Check sheet for the drawn part. Datum: minimum x, y, z corner. Units: mm. A direction names the side the tool comes from. Round coordinates to 2 decimals unless told otherwise and drop trailing zeros. Write each loop counter-clockwise with the first axis right and the second up, starting at its lowest first coordinate (ties: lowest second). Pieces come first, ordered by that corner, then holes. Notation, with made-up numbers: M 63.5,61 L 110.5,61 A8 ccw 110.5,72 Z; hole C 77.25,9.5 d2. An arc over 180 degrees is marked long. Use a Markdown table: item, result.
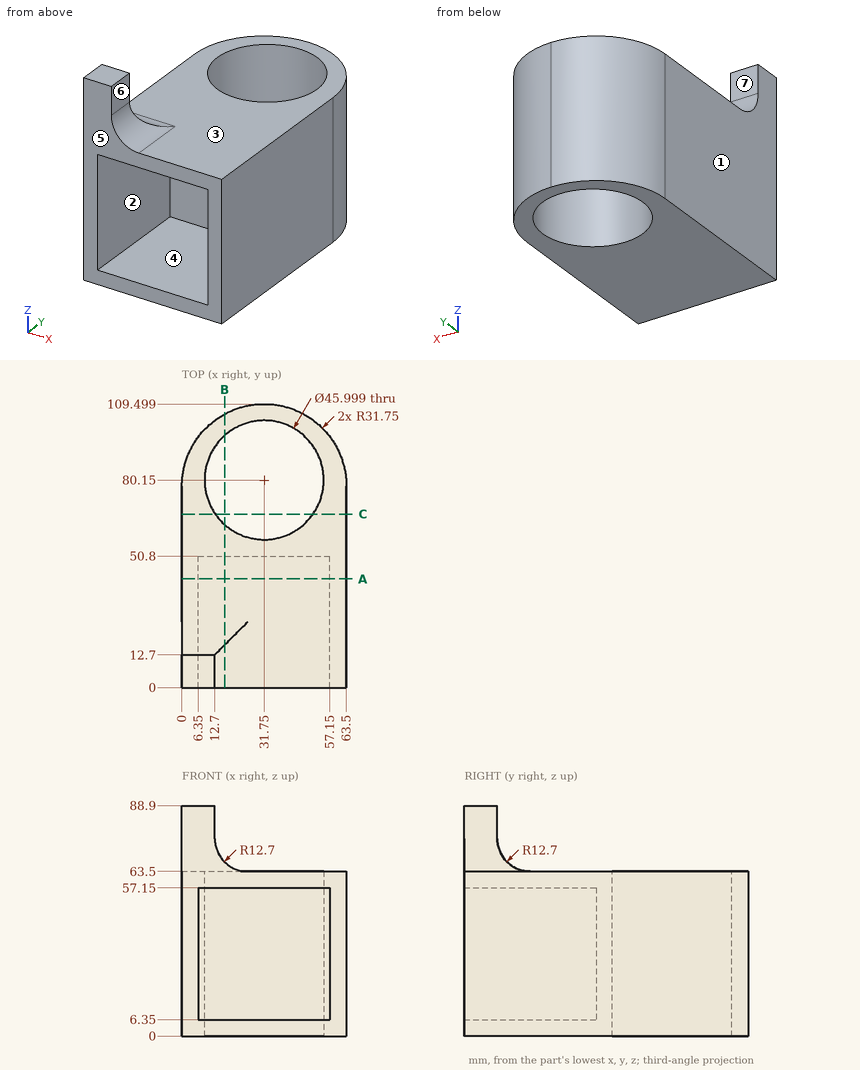
Item 1: Material ranges on line 1 along Y through (x, z) = (31.75, 29); line 2 along Z through (x, y) = (12, 43), recorded low to high. Write a range as from..to.
Outcome:
| item | result |
|---|---|
| line 1 | y = 50.8..57.15, 103.15..109.5 |
| line 2 | z = 0..6.35, 57.15..63.5 |
Item 2: Access from +Z, -Z, +X, -X, +Y, -Y to the whole of each face (thin tool, end or side, straight path). Record for the marked faces 4, 5, 6 and 7.
Outcome:
| item | result |
|---|---|
| face 4 | -Y |
| face 5 | +Z, -Z, +X, -X, -Y |
| face 6 | +Z, +X, +Y, -Y |
| face 7 | +Z, +X, -X, +Y |
Item 3: Go/stop test with flat-tipped pins: pin 1 (5 mm diameter, centred on y = 87, z = 11.5, fed in from -X); pin 2 (4 mm diameter, centred on x = 25.5, y = 44.5, fed in from -Z); pin 3 (10 mm diameter, centred on x = 3, z = 84, fed in from +Y); pin 4 (6 mm diameter, centred on x = 50, y = 28.5, fed in from +Z). Record where each tip stops, or that it passes through.
Outcome:
| item | result |
|---|---|
| pin 1 | stops at x = 0.73 |
| pin 2 | stops at z = 0 |
| pin 3 | stops at y = 12.7 |
| pin 4 | stops at z = 63.5 |
Item 4: Cross-section at B-B, the plane x = 16.5. Record the cut outline in (y, z).
Outcome:
| item | result |
|---|---|
| outline | M 0,0 L 62.93,0 L 62.93,63.5 L 25.4,63.5 A12.7 cw 16.5,67.14 L 0,67.14 L 0,57.15 L 50.8,57.15 L 50.8,6.35 L 0,6.35 Z; M 97.37,0 L 105.6,0 L 105.6,63.5 L 97.37,63.5 Z |
Item 5: Cross-section at C-C, the plane y = 67. Record the cut outline in (x, z).
Outcome:
| item | result |
|---|---|
| outline | M 0,0 L 12.88,0 L 12.88,63.5 L 0,63.5 Z; M 50.62,0 L 63.5,0 L 63.5,63.5 L 50.62,63.5 Z |
Item 6: Cross-section at A-A, the plane y = 42. Record the cut outline in (x, z).
Outcome:
| item | result |
|---|---|
| outline | M 0,0 L 63.5,0 L 63.5,63.5 L 0,63.5 Z; hole M 6.35,6.35 L 57.15,6.35 L 57.15,57.15 L 6.35,57.15 Z |
Item 7: Mould release check, pull along Z, two halves, no side actions. Record for the marked faces 1, 2 and 3: +Z half, -Z half, draft (parallel to the pull), parting line (faces both ways), or undercut.
Outcome:
| item | result |
|---|---|
| face 1 | draft |
| face 2 | undercut |
| face 3 | +Z half |
